from build123d import *

# Parameters (mm, degrees)
SKETCH2_R           = 7.715
BOSS_EXTRUDE1_DEPTH = 21.7
SKETCH4_R           = 1
CUT_EXTRUDE2_DEPTH  = 25.288525068
BOSS_EXTRUDE2_START = 1
SKETCH11_R          = 6.715
BOSS_EXTRUDE2_DEPTH = 1
SKETCH12_R          = 6.715
CUT_EXTRUDE7_DEPTH  = 20.7
CUT_EXTRUDE8_START  = -1
CUT_EXTRUDE8_DEPTH  = 16.275
SKETCH14_W          = 9
SKETCH14_H          = 10.85
CUT_EXTRUDE9_DEPTH  = 52.443281631
FILLET3_R           = 2
FILLET4_R           = 4
CUT_EXTRUDE10_REACH = 30.043
SKETCH15_R          = 1.63


# Read off the part's stored shape, not the designer's step: Cut-Extrude8
with BuildPart() as part:
    # Sketch2 → Boss-Extrude1 (new body)
    with BuildSketch(Plane(origin=(0, 0, 0), x_dir=(1, 0, 0), z_dir=(0, 1, 0))):
        with Locations(Location((0, 0, 0), (0, 0, 270))):
            Circle(SKETCH2_R)
    extrude(amount=BOSS_EXTRUDE1_DEPTH)

    # Sketch4 → Cut-Extrude2 (cut, through all)
    with BuildSketch(Plane(origin=(0, 21.7, 0), x_dir=(1, 0, 0), z_dir=(0, 1, 0))):
        with Locations(Location((0, 0, 0), (0, 0, 270))):
            Circle(SKETCH4_R)
    extrude(amount=-CUT_EXTRUDE2_DEPTH, mode=Mode.SUBTRACT)

    # Sketch11 → Boss-Extrude2 (add)
    with BuildSketch(Plane.XZ.offset(BOSS_EXTRUDE2_START)):
        with BuildLine():
            Line((6.597061846, 4), (16, 4))
            Line((16, 4), (16, -4))
            Line((16, -4), (6.597061846, -4))
            ThreePointArc((6.597061846, -4), (0, -7.715), (-6.597061846, -4))
            Line((-6.597061846, -4), (-16, -4))
            Line((-16, -4), (-16, 4))
            Line((-16, 4), (-6.597061846, 4))
            ThreePointArc((-6.597061846, 4), (0, 7.715), (6.597061846, 4))
        make_face()
        with Locations(Location((0, 0, 0), (0, 0, 270))):
            Circle(SKETCH11_R, mode=Mode.SUBTRACT)
    extrude(amount=-BOSS_EXTRUDE2_DEPTH)

    # Sketch12 → Cut-Extrude7 (cut)
    with BuildSketch(Plane.XZ):
        with Locations(Location((0, 0, 0), (0, 0, 270))):
            Circle(SKETCH12_R)
    extrude(amount=-CUT_EXTRUDE7_DEPTH, mode=Mode.SUBTRACT)

    # Cut-Extrude8 outline → Cut-Extrude8 (cut)
    with BuildSketch(Plane(origin=(0, 0, 0), x_dir=(1, 0, 0), z_dir=(0, 1, 0)).offset(CUT_EXTRUDE8_START)):
        with BuildLine():
            ThreePointArc((4.5, -4.98409721), (0, -6.715), (-4.5, -4.98409721))
            Line((-4.5, -4.98409721), (-4.5, -6.266675754))
            ThreePointArc((-4.5, -6.266675754), (0, -7.715), (4.5, -6.266675754))
            Line((4.5, -6.266675754), (4.5, -4.98409721))
        make_face()
        with BuildLine():
            Line((-4.5, 6.266675754), (-4.5, 4.98409721))
            ThreePointArc((-4.5, 4.98409721), (0, 6.715), (4.5, 4.98409721))
            Line((4.5, 4.98409721), (4.5, 6.266675754))
            ThreePointArc((4.5, 6.266675754), (0, 7.715), (-4.5, 6.266675754))
        make_face()
    extrude(amount=CUT_EXTRUDE8_DEPTH, mode=Mode.SUBTRACT)

    # Sketch14 → Cut-Extrude9 (cut, through all)
    with BuildSketch(Plane(origin=(30, 0, 0), x_dir=(0, 0, -1), z_dir=(1, 0, 0))):
        with Locations((0, 9.85)):
            Rectangle(SKETCH14_W, SKETCH14_H)
    extrude(amount=-CUT_EXTRUDE9_DEPTH, mode=Mode.SUBTRACT)

    # Fillet3
    fillet3_edges = [part.edges().sort_by_distance(p)[0] for p in [
        (4.5, 15.275, 5.625386482),
        (4.5, 15.275, -5.625386482),
        (-4.5, 15.275, -5.625386482),
        (-4.5, 15.275, 5.625386482),
        (5.625386482, 15.275, -4.5),
        (-5.625386482, 15.275, -4.5),
        (5.625386482, 4.425, -4.5),
        (-5.625386482, 4.425, -4.5),
        (-5.625386482, 4.425, 4.5),
        (5.625386482, 4.425, 4.5),
        (5.625386482, 15.275, 4.5),
        (-5.625386482, 15.275, 4.5),
    ]]
    fillet(fillet3_edges, radius=FILLET3_R)

    # Fillet4
    # the kernel refuses this fillet: 4 mm, written as the material it adds along each edge
    with BuildSketch(Plane(origin=(6.597061846, -1, -4), x_dir=(-0.6038984095873641, 0, -0.797061296825942), z_dir=(0, 1, 0)), Plane(origin=(-6.597061846, -1, 4), x_dir=(0.6038984095873637, 0, 0.7970612968259423), z_dir=(0, 1, 0))) as fillet4_piece_1:
        with BuildLine():
            CenterArc((2.003972094, -3.978668209), FILLET4_R, 95.919901586, 46.930484551)
            Line((-1.184273093, -1.563074571), (0, 0))
            ThreePointArc((0, 0), (0.795709969, -0.041143691), (1.591419939, 0))
        make_face()
    extrude(amount=1)
    with BuildSketch(Plane(origin=(6.597061846, -1, 4), x_dir=(-0.6038984095873636, 0, 0.7970612968259423), z_dir=(0, 1, 0)), Plane(origin=(-6.597061846, -1, -4), x_dir=(0.6038984095873643, 0, -0.7970612968259416), z_dir=(0, 1, 0))) as fillet4_piece_2:
        with BuildLine():
            CenterArc((2.003972094, 3.978668209), FILLET4_R, 217.149613863, 46.930484551)
            Line((-1.184273093, 1.563074571), (0, 0))
            ThreePointArc((0, 0), (0.795709969, 0.041143691), (1.591419939, 0))
        make_face()
    extrude(amount=1)
    # the kernel refuses this fillet: 4 mm, written as the material it takes off along each edge
    with BuildSketch(Plane(origin=(16, -11, -4), x_dir=(0, 0, 1), z_dir=(0, 1, 0)), Plane(origin=(16, -11, 4), x_dir=(-1, 0, 0), z_dir=(0, 1, 0))) as fillet4_2_piece_1:
        with BuildLine():
            CenterArc((FILLET4_R, -FILLET4_R), FILLET4_R, 90, 90)
            Line((0, -FILLET4_R), (0, 0))
            Line((0, 0), (FILLET4_R, 0))
        make_face()
    extrude(amount=21, mode=Mode.SUBTRACT)
    with BuildSketch(Plane(origin=(-16, -11, -4), x_dir=(0, 0, 1), z_dir=(0, 1, 0)), Plane(origin=(-16, -11, 4), x_dir=(1, 0, 0), z_dir=(0, 1, 0))) as fillet4_2_piece_2:
        with BuildLine():
            CenterArc((FILLET4_R, FILLET4_R), FILLET4_R, 180, 90)
            Line((0, FILLET4_R), (0, 0))
            Line((0, 0), (FILLET4_R, 0))
        make_face()
    extrude(amount=21, mode=Mode.SUBTRACT)

    # Sketch15 → Cut-Extrude10 (cut, up to next)
    with BuildSketch(Plane(origin=(0, 0, 0), x_dir=(1, 0, 0), z_dir=(0, 1, 0)), mode=Mode.PRIVATE) as cut_extrude10_sk1:
        with Locations(Location((-12, 0, 0), (0, 0, 270))):
            Circle(SKETCH15_R)
    cut_extrude10_tool1 = extrude(cut_extrude10_sk1.sketch, amount=-CUT_EXTRUDE10_REACH, mode=Mode.PRIVATE) & part.part
    # Sketch15 → Cut-Extrude10 (cut, up to next)
    with BuildSketch(Plane(origin=(0, 0, 0), x_dir=(1, 0, 0), z_dir=(0, 1, 0)), mode=Mode.PRIVATE) as cut_extrude10_sk2:
        with Locations(Location((12, 0, 0), (0, 0, 270))):
            Circle(SKETCH15_R)
    cut_extrude10_tool2 = extrude(cut_extrude10_sk2.sketch, amount=-CUT_EXTRUDE10_REACH, mode=Mode.PRIVATE) & part.part
    add(cut_extrude10_tool1.solids().sort_by_distance((-12, 0, 0))[0], mode=Mode.SUBTRACT)
    add(cut_extrude10_tool2.solids().sort_by_distance((12, 0, 0))[0], mode=Mode.SUBTRACT)


solid = part.part
Work out the finished part from the listing and answer in its coordinate system (mm). A direction names the side the tool comes from. Coordinates: 2 decimals unless noted, no trailing zeros. Loops run counter-clockwise (first coordinate to the right, second up) from the corner with the lowest first, then second, coordinate; pieces in that order, holes last. Notation, with made-up numbers: (1.5, -14.5) -> (14.5, -14.5) arc R13 ccw to (14.5, 8.5) -> close; hole circle Ø6 at (-27.5, 53.5). An arc over 180 degrees is marked (long way). Write each question's results on one line, items separated by ' | '. Start each with the question number.
1) For faces 4 (the cylindrical face through (4.54, 14.52, 4.95)), 5 (the flat face through (-4.5, 6, -6)), 6 (the flat face through (7, 4.425, 0)), determine the directions among +Z, -Z, +X, -X, +Y, -Y from which every point of the face is accessible in a straight line to the end or side of a thin tool.
2) Flat-ended cylindrical pins translate along their axes: P1, Ø6.5, axis at x = 2, z = 2, coming from the -Y side; P2, Ø1, axis at x = 5.5, y = 10.5, coming from the +Z side; P3, Ø1.5, axis at x = -3, y = 11, coming from the -Z side; P4, Ø1.5, axis at x = 9.5, z = -2.5, coming from the +Y side. Find the tip coordinate at first contact, or state that the pin passes through.
3) Find section D-D on z = 2. Determine the outline of the cut face in (x, y) (3 decimals), then the cut area to 3 significant figures.
4) Find section C-C on y = 2.5. Determine the outline of the cut face in (x, z) (3 decimals), then the cut area to 3 significant figures.
5) Find section B-B on z = 0. Count the separate pieces of the cut face and the enclosed holes in it, then the cut area to 3 significant figures.
6) Find section A-A on x = 0. Determine the outline of the cut face in (y, z) (3 decimals).
7) The mould has two halves that part along Z. Classify faces 1 (the cylindrical face through (6.99, -0.51, 4.32)), 2 (the flat face through (0, 15.275, -7)), 3 (the cylindrical face through (6.125, 5.026, -3.93)): pulls with the +Z half, pulls with the -Z half, needs draft (parallel to the pull), parting line crosses it, or undercut.
8) Consider line 1 along Z through (x, y) = (-4.5, 13.75); line 2 along X through (y, z) = (3.25, 2.5). Determine where each line is inside the solid, lowest interval first.
Response values:
1) face 4: -Y | face 5: +Z, -Z, -Y | face 6: +X, -X
2) P1: stops at y = 20.7 | P2: stops at z = 5.88 | P3: passes through | P4: stops at y = 0
3) outline: (-15.464, -1) -> (-6.41, -1) -> (-6.41, 4.425) -> (-7.451, 4.425) -> (-7.451, 0) -> (-15.464, 0) -> close; (-7.451, 15.275) -> (-6.41, 15.275) -> (-6.41, 20.7) -> (6.41, 20.7) -> (6.41, 15.275) -> (7.451, 15.275) -> (7.451, 21.7) -> (-7.451, 21.7) -> close; (6.41, -1) -> (15.464, -1) -> (15.464, 0) -> (7.451, 0) -> (7.451, 4.425) -> (6.41, 4.425) -> close | area: 53.5 mm^2
4) outline: (-4.5, -6.267) -> (-4.5, -4.984) arc R6.715 cw to (-4.5, 4.984) -> (-4.5, 6.267) arc R7.715 ccw to start; (4.5, -6.267) arc R7.715 ccw to (4.5, 6.267) -> (4.5, 4.984) arc R6.715 cw to (4.5, -4.984) -> close | area: 25.9 mm^2
5) separate pieces: 6 | enclosed holes: 0 | area: 45.2 mm^2
6) outline: (15.275, -7.715) -> (21.7, -7.715) -> (21.7, -1) -> (20.7, -1) -> (20.7, -6.715) -> (15.275, -6.715) -> close; (15.275, 6.715) -> (20.7, 6.715) -> (20.7, 1) -> (21.7, 1) -> (21.7, 7.715) -> (15.275, 7.715) -> close
7) face 1: pulls with the +Z half | face 2: needs draft | face 3: undercut
8) line 1: z = -6.27 to -4.98, 4.98 to 6.27 | line 2: x = -7.3 to -6.23, 6.23 to 7.3
